Source: three-view drawing plus pictorial views. Frame: mm from the lowest corner of the part. Coordinates: 2 decimals unless noted, no trailing zeros. One line per question, with ' | ' between items.
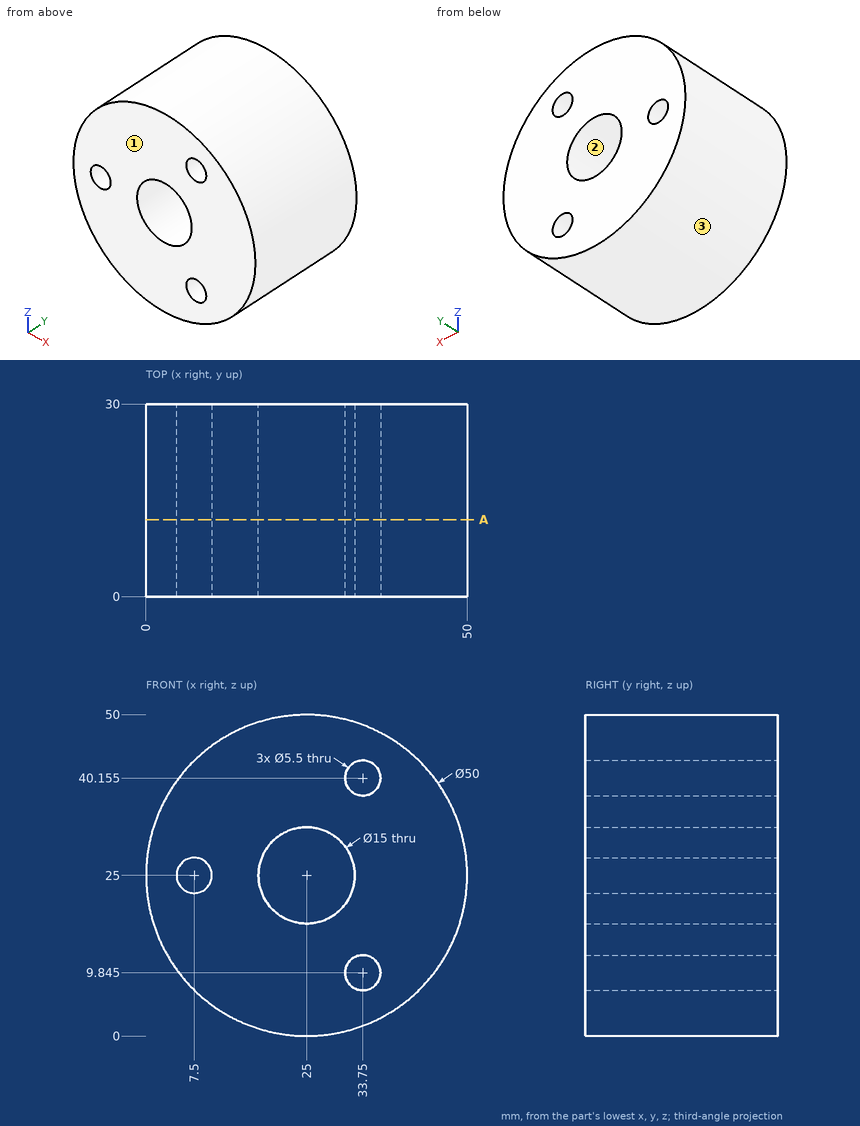
1. Material intervals for line 1 (X direction, y = 17, z = 25); line 2 (Z direction, x = 25, y = 24); line 3 (Z direction, x = 33, y = 2.5) (1 decimal), sorted ascending. Write a range as [from, to].
Response values:
line 1: x = [0, 4.75], [10.25, 17.5], [32.5, 50] | line 2: z = [0, 17.5], [32.5, 50] | line 3: z = [1.3, 7.2], [12.5, 37.5], [42.8, 48.7]
2. Section A-A, the plane y = 12. Give the number of separate pieces and of enclosed holes in the cut face, and give its area (3 significant figures).
Response values:
separate pieces: 1 | enclosed holes: 4 | area: 1,720 mm^2
3. Draft query along X for the marked faces 1, 2 and 3. Return one class per face: pulls with the +X half, pulls with the -X half, needs draft (parallel to the pull), parting line crosses it, or undercut.
Response values:
face 1: needs draft | face 2: undercut | face 3: parting line crosses it
4. Pin query (flat end, axial travel): P1, Ø9, axis at x = 25, z = 25, coming from the +Y side (3 decimals); P2, Ø1.5, axis at y = 19.5, z = 37.5, coming from the -X side; P3, Ø1, axis at y = 13, z = 13, coming from the +X side; P4, Ø2, axis at y = 19.5, z = 11, coming from the -X side (1 decimal). Return the tip coordinate at first contact, or that it passes through.
Response values:
P1: passes through | P2: stops at x = 2.93 | P3: stops at x = 47.2 | P4: stops at x = 3.6
